Study the drawing (mm; zero at the part's minimum x, y, z) and answer. Give positions to 0.01 mm unless a question says otherwise; leave off trailing zeros. Order: outer loops, then holes, each group sorted by start corner. A loop starts at its lowest first (then second) coordinate and runs counter-clockwise, first axis right, second up. Notation, with made-up numbers: (12, 13.25) - (40, 13.25) arc R8 ccw to (40, 20.25) - close; hole circle Ø1 at (-38, -7.75). An arc over 180 degrees is marked (long way). Write each question's results on one line, items separated by ' | '. Start each with the question number.
1. Section A-A (z = 4.5) is taken. Give the vertices of the cut face in (x, y) (1 decimal).
2. Flat-ended cylindrical pins translate along their axes: pin 1 (1.5 mm diameter, centred on y = 124, z = 7.5, fed in from -X) (1 decimal); pin 2 (1 mm diameter, centred on y = 106, z = 2.5, fed in from -X) (1 decimal); pin 3 (5 mm diameter, centred on x = 59, z = 4, fed in from +Y) (1 decimal). Find the tip coordinate at first contact, or state that the pin passes through.
3. Section B-B (y = 5) is taken. Give the vertices of the cut face in (x, z).
4. Find the intervals of material crossed by L1, parallel to Y at x = 41, z = 5 (1 decimal); L2, parallel to Y at x = 81, z = 7.5 (1 decimal); L3, parallel to Y at x = 206, z = 7, in increasing order.
5. Section C-C (x = 187) is taken. Give the vertices of the cut face in (y, z).
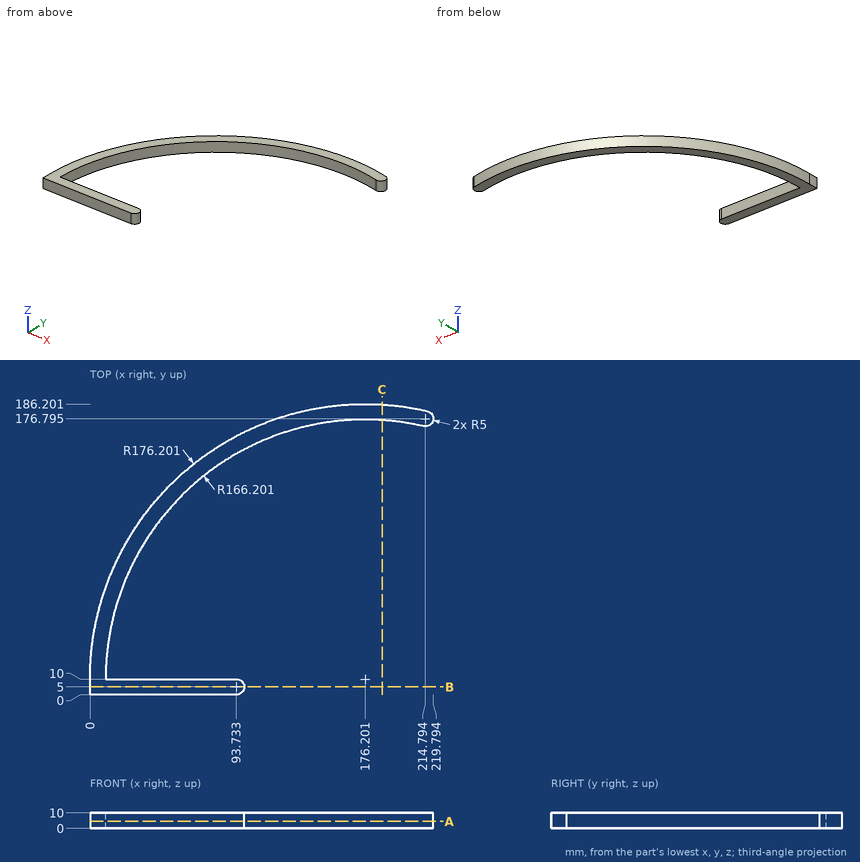
Reported:
1) outline: (0, 0) - (93.7, 0) arc R5 ccw to (93.7, 10) - (10, 10) arc R166.2 cw to (213.7, 171.9) arc R5 ccw to (215.9, 181.7) arc R176.2 ccw to (0, 10) - close
2) pin 1: x = 41.2 | pin 2: x = 28.1 | pin 3: y = 143.8
3) outline: (0, 0) - (98.73, 0) - (98.73, 10) - (0, 10) - close
4) L1: 0 to 10, 106.7 to 123 | L2: 0 to 10, 146.2 to 158.3 | L3: 173.51 to 183.66
5) outline: (175.85, 0) - (185.87, 0) - (185.87, 10) - (175.85, 10) - close
